Can you work these out from the drawing? Everything is in mm from the part's minimum corner. A direction names the side the tool comes from. Coordinates: 2 decimals unless noted, no trailing zeros. Write each loop counter-clockwise with the first axis right and the second up, starting at its lowest first coordinate (ties: lowest second). Pieces come first, ordered by that corner, then holes. Notation, with made-up numbers: (52, 65) -> (63, 65) arc R8 ccw to (63, 71) -> close; hole circle Ø9 at (67, 73). An arc over 180 degrees is marked (long way). Answer as CSV lines item,"result". Start each with the question number.
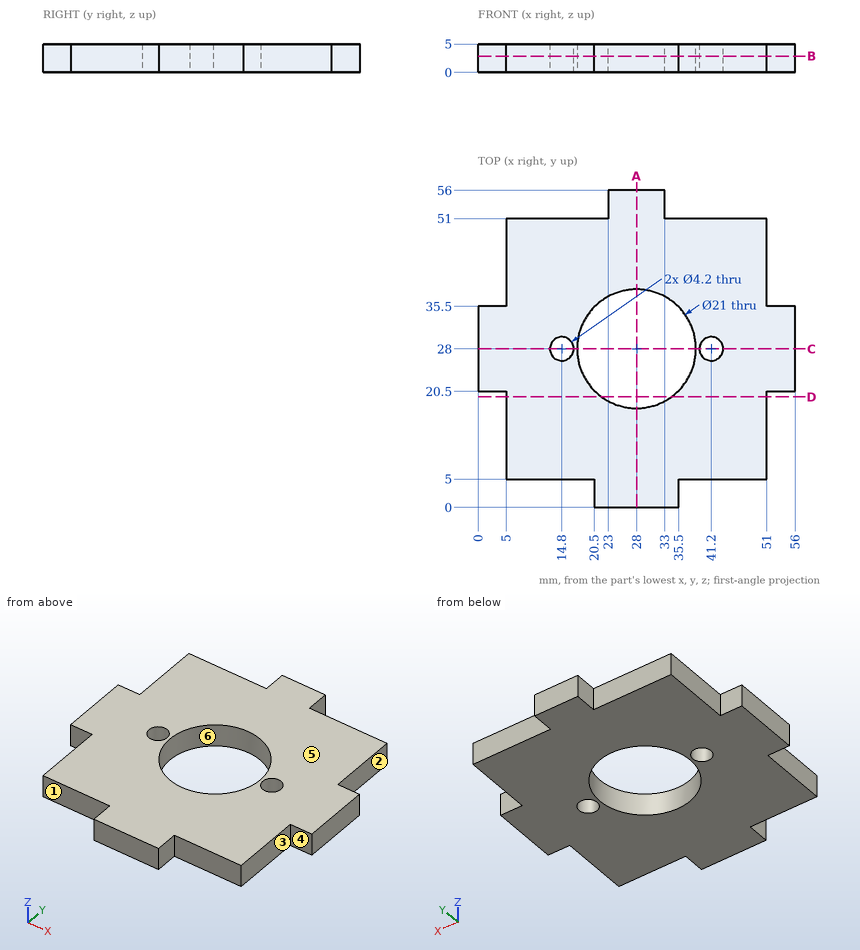
Q1. Which directions (+Z, -Z, +X, -X, +Y, -Y) give clear straight access to the entire face, cutting with the end or side of a thin tool? Please do the marked faces 1, 2 and 3.
Q2. Imagine slicing it at D-D (y = 19.5). Write out the boundary of the cut face in (x, z).
Q3. I need wall thicknesses on L1, parallel to Y at x = 27.5, z = 0.85; L2, parallel to Y at x = 14.8, z = 3.55; L3, parallel to Y at x = 44, z = 0.2. Which ranges of each line are inside material? Lowest first, please.
Q4. Imagine slicing it at B-B (z = 2.85). Write out the boundary of the cut face in (x, y).
Q5. If we mould it in two halves opening along Y, with no side actions, what happens to the marked faces 4, 5 and 6? For each: released by +Y, released by -Y, zero draft, split by the parting line, or undercut.
Q6. Imagine slicing it at A-A (x = 28). Write out the boundary of the cut face in (y, z).
Q7. Imagine slicing it at C-C (y = 28). Write out the boundary of the cut face in (x, z), then the cut area to 3 significant figures.
Q8. For pin 1 (1.5 mm diameter, centred on y = 1.5, z = 1.5, fed in from -X); pin 2 (1.5 mm diameter, centred on y = 54, z = 3.5, fed in from +X); pin 3 (2.5 mm diameter, centred on x = 3, z = 3.5, fed in from -Y); pin 4 (2.5 mm diameter, centred on x = 41.2, y = 28, fed in from +Z), each with a flat end and sliding along its axis, tell me the tip position at first contact or that it passes through.
Entries:
1,face 1,"+Z, -Z, -X, -Y"
1,face 2,"+Z, -Z, +X, +Y"
1,face 3,"+Z, -Z, +X, -Y"
2,outline,"(5, 0) -> (21.84, 0) -> (21.84, 5) -> (5, 5) -> close; (34.16, 0) -> (51, 0) -> (51, 5) -> (34.16, 5) -> close"
3,L1,"0 to 17.51, 38.49 to 56"
3,L2,"5 to 25.9, 30.1 to 51"
3,L3,"5 to 51"
4,outline,"(0, 20.5) -> (5, 20.5) -> (5, 5) -> (20.5, 5) -> (20.5, 0) -> (35.5, 0) -> (35.5, 5) -> (51, 5) -> (51, 20.5) -> (56, 20.5) -> (56, 35.5) -> (51, 35.5) -> (51, 51) -> (33, 51) -> (33, 56) -> (23, 56) -> (23, 51) -> (5, 51) -> (5, 35.5) -> (0, 35.5) -> close; hole circle Ø4.2 at (14.8, 28); hole circle Ø21 at (28, 28); hole circle Ø4.2 at (41.2, 28)"
5,face 4,"released by -Y"
5,face 5,"zero draft"
5,face 6,"undercut"
6,outline,"(0, 0) -> (17.5, 0) -> (17.5, 5) -> (0, 5) -> close; (38.5, 0) -> (56, 0) -> (56, 5) -> (38.5, 5) -> close"
7,outline,"(0, 0) -> (12.7, 0) -> (12.7, 5) -> (0, 5) -> close; (16.9, 0) -> (17.5, 0) -> (17.5, 5) -> (16.9, 5) -> close; (38.5, 0) -> (39.1, 0) -> (39.1, 5) -> (38.5, 5) -> close; (43.3, 0) -> (56, 0) -> (56, 5) -> (43.3, 5) -> close"
7,area,"133 mm2"
8,pin 1,"x = 20.5"
8,pin 2,"x = 33"
8,pin 3,"y = 20.5"
8,pin 4,"through"
